Could you check a few things on this model? Use its own coordinates, in mm. A direction names the side the tool comes from. Coordinates: 2 decimals unless noted, no trailing zeros. Write each loop counter-clockwise with the first axis right and the second up, starting at its lowest first coordinate (ties: lowest second). Pieces come first, ordered by that corner, then holes.
```python
from build123d import *

# Parameters (mm, degrees)
F1_DEPTH = 26
F2_R     = 11.2
F3_DEPTH = 25
F5_DEPTH = 2
F7_DEPTH = 7


with BuildPart() as f1:
    # F0 (on Top) → F1 (new body)
    with BuildSketch(Plane.XY):
        with BuildLine():
            ThreePointArc((13, 17.748239), (20.54045, 7.879715), (21.534855, -4.5))
            Line((21.534855, -4.5), (24.591665, -4.5))
            Line((24.591665, -4.5), (24.591665, 4.5))
            ThreePointArc((24.591665, 4.5), (10.227772, 22.812117), (-13, 21.354157))
            Line((-13, 21.354157), (-13, 14))
            Line((-13, 14), (13, 14))
            Line((13, 14), (13, 17.748239))
        make_face()
    extrude(amount=F1_DEPTH)

    # F2 (on face) → F3 (cut)
    with BuildSketch(Plane.XZ.offset(-14)):
        with Locations((0, 13)):
            Circle(F2_R)
    extrude(amount=-F3_DEPTH, mode=Mode.SUBTRACT)

    # F4 (on face) → F5 (join)
    with BuildSketch(Plane.YZ.offset(24.591665)):
        with BuildLine():
            ThreePointArc((-4.5, 13), (0, 8.5), (4.5, 13))
            ThreePointArc((4.5, 13), (0, 17.5), (-4.5, 13))
        make_face()
    extrude(amount=F5_DEPTH)

    # F6 (on face) → F7 (join)
    with BuildSketch(Plane.YZ.offset(26.591665)):
        with BuildLine():
            ThreePointArc((0.5, 9.535898), (3.5, 13), (0.5, 16.464102))
            Line((0.5, 16.464102), (0.5, 13.866025))
            ThreePointArc((0.5, 13.866025), (1, 13), (0.5, 12.133975))
            Line((0.5, 12.133975), (0.5, 9.535898))
        make_face()
        with BuildLine():
            Line((-0.5, 13.866025), (-0.5, 16.464102))
            ThreePointArc((-0.5, 16.464102), (-3.5, 13), (-0.5, 9.535898))
            Line((-0.5, 9.535898), (-0.5, 12.133975))
            ThreePointArc((-0.5, 12.133975), (-1, 13), (-0.5, 13.866025))
        make_face()
    extrude(amount=F7_DEPTH)


solid = f1.part
```
1. I want a section at C-C on z = 2.5. Please give me the cut outline in (x, y), plus the area to 3 significant figures.
Verdict:
outline: (-13, 14) - (-3.9, 14) - (-3.9, 24.69) arc R25 ccw to (-13, 21.35) - close; (3.9, 14) - (13, 14) - (13, 17.75) arc R22 cw to (21.53, -4.5) - (24.59, -4.5) - (24.59, 4.5) arc R25 ccw to (3.9, 24.69) - close
area: 251 mm2
2. I want a section at B-B on x = 0. Please give me the cut outline in (y, z).
Verdict:
outline: (14, 0) - (25, 0) - (25, 1.8) - (14, 1.8) - close; (14, 24.2) - (25, 24.2) - (25, 26) - (14, 26) - close
3. I want a section at D-D on y = 0. Please give me the cut outline in (x, z), plus the area to 3 significant figures.
Verdict:
outline: (22, 0) - (24.59, 0) - (24.59, 8.5) - (26.59, 8.5) - (26.59, 17.5) - (24.59, 17.5) - (24.59, 26) - (22, 26) - close
area: 85.4 mm2
4. On a 3-axis mill with a long thin cutter (end or side, diameter ignored), from which of +Z, -Z, +X, -X, +Y, -Y can I reach the whole of each face in a straight line? I mean faces 1 (the face through (13, 16, 13)), 2 (the face through (25.578, 2.419, 16.794)), 3 (the face through (-12, 14, 13)), 4 (the face through (30, -3.5, 13.1)). Say none if no direction works.
Verdict:
face 1: +Z, -Z, -Y
face 2: +X
face 3: +Z, -Z, -X, -Y
face 4: +X, -Y
5. If we mould it in two halves opening along Y, with no side actions, what happens to faces 5 (the face through (30, 1, 13)), 6 (the face through (23, -4.5, 13)), 7 (the face through (30, 3.5, 12.9))? For each: pulls with the +Y half, pulls with the -Y half, needs draft (parallel to the pull), parting line crosses it, or undercut.
Verdict:
face 5: undercut
face 6: pulls with the -Y half
face 7: pulls with the +Y half
6. For pin 1 (3 mm diameter, centred on x = 30, z = 11, fed in from -Y); pin 2 (3 mm diameter, centred on x = 28.5, z = 15.5, fed in from +Y); pin 3 (1.5 mm diameter, centred on x = 8.5, z = 6, fed in from -Y); pin 4 (13.5 mm diameter, centred on x = 0, z = 13, fed in from -Y), each with a flat end and sliding along its axis, tell me the tip position at first contact or that it passes through.
Verdict:
pin 1: stops at y = -3.46
pin 2: stops at y = 3.35
pin 3: stops at y = 14
pin 4: passes through
7. Please list where these lines run through material, in increasing order: line 1 along Z through (x, y) = (0, 19.75); line 2 along X through (y, z) = (20, 13); line 3 along Y through (x, z) = (28, 10.5).
Verdict:
line 1: z = 0 to 1.8, 24.2 to 26
line 2: x = -13 to -11.2, 11.2 to 15
line 3: y = -2.45 to -0.5, 0.5 to 2.45
8. I want a section at A-A on y = 15. Please give me the cut outline in (x, z), plus the area to 3 significant figures.
Verdict:
outline: (-13, 0) - (13, 0) - (13, 26) - (-13, 26) - close; (16.09, 0) - (20, 0) - (20, 26) - (16.09, 26) - close; hole circle Ø22.4 at (0, 13)
area: 383 mm2
